Could you check a few things on this model? Use its own coordinates, in mm. A direction names the side the tool comes from. Give positions to 0.01 mm unless a question says otherwise; leave off trailing zeros. Loops run counter-clockwise (first coordinate to the right, second up) from the corner with the lowest first, then second, coordinate; pieces in that order, holes last. Notation, with made-up numbers: (-18.5, -20) -> (40.5, -20) arc R12 cw to (40.5, -12) -> close; hole circle Ø3 at (69.25, 79.25). An arc over 180 degrees is marked (long way). Put each result on its own line as item: value.
```python
from build123d import *

# Parameters (mm, degrees)
F1_DEPTH = 19.05


with BuildPart() as f1:
    # F0 (on Top) → F1 (new body)
    with BuildSketch(Plane.XY):
        Polygon((127.374873, 0), (130.079165, 0), (283.87782, 0), (286.131769, 18.14894), (281.604767, 26.116442), (281.604767, 30.82451), (278.164268, 36.981218), (278.164268, 41.146047), (279.43182, 48.751391), (281.242609, 52.735142), (281.242609, 60.883723), (289.029032, 82.251117), (291.432261, 110.667914), (298.728049, 116.189055), (298.728049, 126.121819), (297.107786, 132.371083), (302.621841, 143.031597), (307.216913, 147.99425), (309.054911, 156.63293), (316.406995, 164.720222), (316.406995, 170.969486), (320.634454, 173.175111), (320.634454, 176.851138), (325.413287, 179.975778), (325.413287, 185.26645), (329.513514, 189.175025), (329.513514, 192.59502), (321.59701, 192.59502), (316.711307, 185.26645), (312.314153, 176.227897), (305.962741, 168.166474), (296.191305, 159.86076), (288.129896, 149.356484), (277.137041, 142.760769), (269.075632, 136.165068), (271.274179, 145.692199), (274.694204, 153.997913), (280.312747, 160.593614), (283.732742, 167.18933), (291.794181, 171.342179), (295.214176, 177.693605), (290.902208, 180.015432), (287.152767, 182.090744), (287.152767, 186.732173), (290.328473, 192.59502), (290.328473, 198.457882), (281.534195, 195.282161), (277.381331, 198.213592), (282.837977, 205.943848), (281.40533, 220.303819), (262.460262, 227.495939), (262.460262, 230.302602), (265.793204, 236.091375), (223.517641, 242.757231), (154.819116, 263.218462), (149.376005, 273.818195), (122.446977, 285.277367), (113.852613, 280.69371), (108.695991, 280.69371), (115.571484, 288.142145), (112.78723, 290.71223), (121.705609, 300.373787), (112.993173, 302.752584), (95.231473, 297.022998), (88.642456, 292.152852), (72.02667, 289.001584), (44.238199, 289.001584), (34.797754, 284.43718), (34.797754, 245.544836), (30.27996, 242.009178), (13.190903, 232.973576), (9.448506, 224.560991), (3.278016, 217.509001), (0, 210.457027), (9.889254, 210.457027), (16.500488, 200.760543), (10.109629, 191.945568), (10.109629, 152.718902), (21.735432, 143.29727), (35.956949, 139.817506), (35.956949, 133.20598), (55.791546, 127.290398), (60.663197, 114.41531), (87.10932, 100.14832), (92.637829, 91.069408), (95.655568, 62.981203), (101.226784, 62.981203), (101.226784, 56.945719), (104.940929, 53.463712), (104.940929, 50.678104), (97.048372, 42.089149), (101.226784, 26.071908), (105.637327, 14.697347), (121.170625, 10.366562), align=None)
    extrude(amount=F1_DEPTH)


solid = f1.part
```
1. I need wall thicknesses on line 1 (X direction, y = 173.5, z = 10); line 2 (Y direction, x = 263, z = 15.5); line 3 (X direction, y = 149, z = 11). Which ranges of each line are inside material? Lowest first, please.
Recorded:
line 1: x = 10.11 to 292.96, 310.16 to 320.63
line 2: y = 0 to 227.29, 231.24 to 236.53
line 3: x = 14.7 to 272.64, 287.54 to 307.43
2. Thinking about a two-plate mould opening in Y: for faces 5 (the face through (112.09, 284.37, 9.39)), 6 (the face through (11.346, 228.826, 9.392)), 7 (the face through (113.3, 12.56, 9.39)), which applies, pulls with the +Y half, pulls with the -Y half, needs draft (parallel to the pull), parting line crosses it, or undercut?
Recorded:
face 5: undercut
face 6: pulls with the +Y half
face 7: pulls with the -Y half
3. I'm going to push flat-ended pins straight in: pin 1 (1 mm diameter, centred on y = 137, z = 10, fed in from -X); pin 2 (2.5 mm diameter, centred on y = 183.5, z = 10, fed in from +X); pin 3 (2 mm diameter, centred on y = 39, z = 12, fed in from +X). Where does each tip first touch, or does it pass through?
Recorded:
pin 1: stops at x = 35.96
pin 2: stops at x = 325.41
pin 3: stops at x = 278.16
4. If we section it at A-A (y = 71): List the corners of the cut face in (x, z) for me.
Recorded:
outline: (94.79, 0) -> (284.93, 0) -> (284.93, 19.05) -> (94.79, 19.05) -> close
5. If we section it at B-B (x = 161.5): List the corners of the cut face in (y, z) for me, then the cut area to 3 significant figures.
Recorded:
outline: (0, 0) -> (261.23, 0) -> (261.23, 19.05) -> (0, 19.05) -> close
area: 4,980 mm^2
6. For faces 1 (the face through (292.217, 154.682, 9.392)), 2 (the face through (272.065, 223.85, 9.392)), 3 (the face through (13.149, 205.677, 9.392)), 4 (the face through (309.18, 172.25, 9.39)), which set-ups out of +Z, -Z, +X, -X, +Y, -Y let a thin tool reach every point of the face, with its end or its side?
Recorded:
face 1: +Z, -Z
face 2: +Z, -Z, +X
face 3: +Z, -Z, -X
face 4: +Z, -Z, +Y
